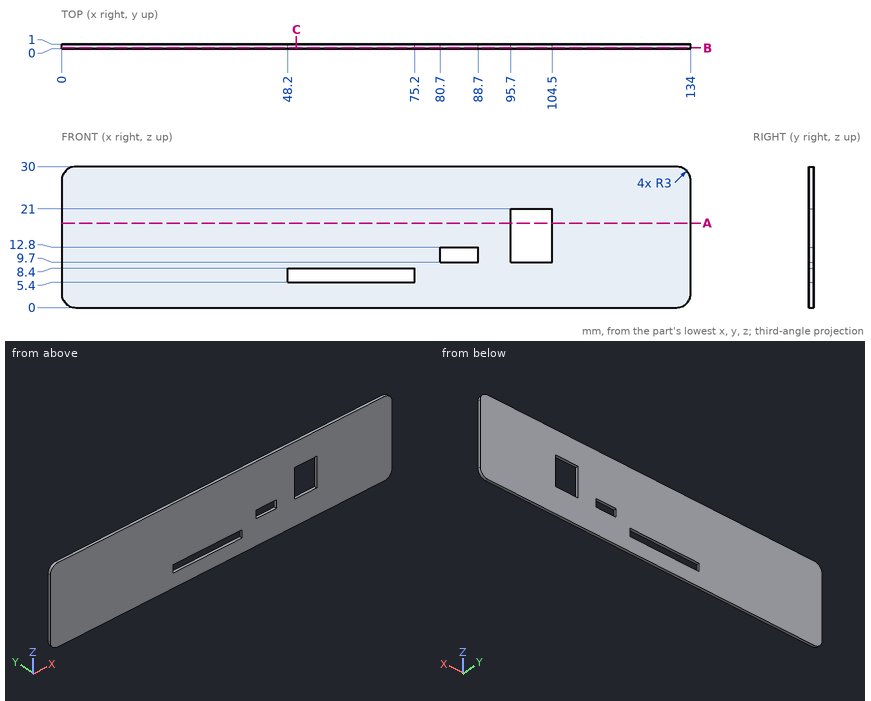
Check sheet for the drawn part. Datum: minimum x, y, z corner. Units: mm. Round coordinates to 2 decimals unless told otherwise and drop trailing zeros. Loops run counter-clockwise (first coordinate to the right, second up) from the corner with the lowest first, then second, coordinate; pieces in that order, holes last. Notation, with made-up numbers: (4, 23) -> (57, 23) arc R26 ccw to (57, 58) -> close; hole circle Ø4 at (50.25, -17.75). An arc over 180 degrees is marked (long way). Put each result on its own line as item: value. Start each with the question number.
1. Scan lines: probe 1 along X at (y, z) = (0.65, 16); probe 2 along Z at (x, y) = (99, 0.6); probe 3 along Z at (x, y) = (75, 0.35). Record each from-to range of solid material in increasing order.
2. Section check A-A (z = 18). Enter the section's corners in (x, y), plus the area to 3 significant figures.
3. Section check C-C (x = 50). Enter the section's corners in (y, z), plus the area to 3 significant figures.
4. Section check B-B (y = 0.15). Enter the section's corners in (x, z).
Findings:
1. probe 1: x = 0 to 95.7, 104.5 to 134
1. probe 2: z = 0 to 9.7, 21 to 30
1. probe 3: z = 0 to 5.4, 8.4 to 30
2. outline: (0, 0) -> (95.7, 0) -> (95.7, 1) -> (0, 1) -> close; (104.5, 0) -> (134, 0) -> (134, 1) -> (104.5, 1) -> close
2. area: 125 mm^2
3. outline: (0, 0) -> (1, 0) -> (1, 5.4) -> (0, 5.4) -> close; (0, 8.4) -> (1, 8.4) -> (1, 30) -> (0, 30) -> close
3. area: 27.0 mm^2
4. outline: (0, 3) arc R3 ccw to (3, 0) -> (131, 0) arc R3 ccw to (134, 3) -> (134, 27) arc R3 ccw to (131, 30) -> (3, 30) arc R3 ccw to (0, 27) -> close; hole (48.2, 5.4) -> (75.2, 5.4) -> (75.2, 8.4) -> (48.2, 8.4) -> close; hole (80.7, 9.7) -> (88.7, 9.7) -> (88.7, 12.8) -> (80.7, 12.8) -> close; hole (95.7, 9.7) -> (104.5, 9.7) -> (104.5, 21) -> (95.7, 21) -> close
